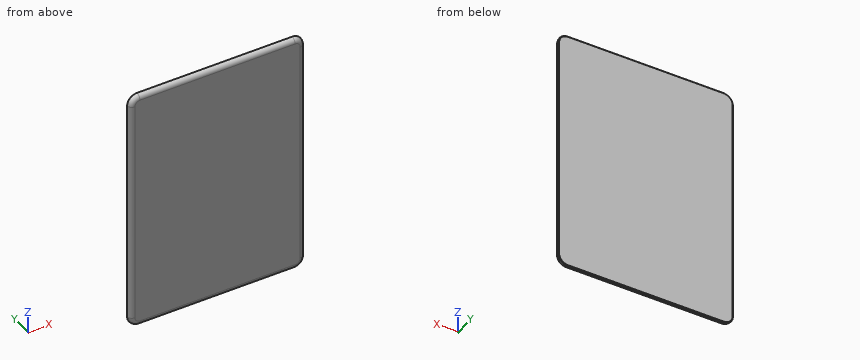
```python
from build123d import *

# Parameters (mm, degrees)
F1_DEPTH = 6.9
F2_R     = 6
F3_SIZE  = 0.89999


# Not quite as in the source:
# - a fillet or chamfer is up to 0.001 mm smaller than in the source, because OpenCascade refuses the exact size


with BuildPart() as f1:
    # F0 (on Front) → F1 (new body)
    with BuildSketch(Plane.XZ):
        with BuildLine():
            Line((97.8, 152.85), (-97.8, 152.85))
            ThreePointArc((-97.8, 152.85), (-106.6388347648, 149.1888347648), (-110.3, 140.35))
            Line((-110.3, 140.35), (-110.3, -140.35))
            ThreePointArc((-110.3, -140.35), (-106.6388347648, -149.1888347648), (-97.8, -152.85))
            Line((-97.8, -152.85), (97.8, -152.85))
            ThreePointArc((97.8, -152.85), (106.6388347648, -149.1888347648), (110.3, -140.35))
            Line((110.3, -140.35), (110.3, 140.35))
            ThreePointArc((110.3, 140.35), (106.6388347648, 149.1888347648), (97.8, 152.85))
        make_face()
    extrude(amount=F1_DEPTH)

    # F2
    f2_edges = [f1.edges().sort_by_distance(p)[0] for p in [
        (110.3, -6.9, 0),
        (106.638835, -6.9, 149.188835),
        (0, -6.9, 152.85),
        (-106.638835, -6.9, 149.188835),
        (-110.3, -6.9, 0),
        (-106.638835, -6.9, -149.188835),
        (0, -6.9, -152.85),
        (106.638835, -6.9, -149.188835),
    ]]
    fillet(f2_edges, radius=F2_R)

    # F3 (size 0.9 in the source; OpenCascade refuses exactly that, so slightly less here)
    f3_edges = [f1.edges().sort_by_distance(p)[0] for p in [
        (110.3, 0, 0),
        (106.638835, 0, 149.188835),
        (0, 0, 152.85),
        (-106.638835, 0, 149.188835),
        (-110.3, 0, 0),
        (-106.638835, 0, -149.188835),
        (0, 0, -152.85),
        (106.638835, 0, -149.188835),
    ]]
    chamfer(f3_edges, length=F3_SIZE)


solid = f1.part
```
Can you work these out from the model? Positions are in its coordinate system, mm. Coordinates: 2 decimals unless noted, no trailing zeros. Loops run counter-clockwise (first coordinate to the right, second up) from the corner with the lowest first, then second, coordinate; pieces in that order, holes last. Notation, with made-up numbers: (17, -6) -> (27, -6) arc R26 cw to (27, 31) -> close; hole circle Ø4 at (26, -38.5). An arc over 180 degrees is marked (long way). Answer as a JSON object with one key per item and string values.
1) If I drill on line 1 (Z direction, x = -81.5, y = -1.5); line 2 (X direction, y = -1, z = 1.5); line 3 (X direction, y = -2.75, z = 134.5), over which ranges is the centre line in solid material (lowest first)?
Results:
{"line 1": "z = -152.82 to 152.82", "line 2": "x = -110.3 to 110.3", "line 3": "x = -110.01 to 110.01"}
2) Imagine slicing it at A-A (y = -5.75). Please give me the cut outline in (x, z), then the cut area to 3 significant figures.
Results:
{"outline": "(-107.83, -140.35) arc R10.03 ccw to (-97.8, -150.38) -> (97.8, -150.38) arc R10.03 ccw to (107.83, -140.35) -> (107.83, 140.35) arc R10.03 ccw to (97.8, 150.38) -> (-97.8, 150.38) arc R10.03 ccw to (-107.83, 140.35) -> close", "area": "64,800 mm^2"}
3) For P1, Ø1.5, axis at x = -78.5, y = -5, coming from the -Z side, with a flat end and sliding along its axis, tell me the tip position at first contact or that it passes through.
Results:
{"P1": "stops at z = -151.83"}
